For this review, take the finished solid that the model builds, in its own axes (mm). Round coordinates to 2 decimals unless told otherwise and drop trailing zeros. Write each loop counter-clockwise with the first axis right and the second up, starting at its lowest first coordinate (ties: lowest second). Pieces come first, ordered by that corner, then holes.
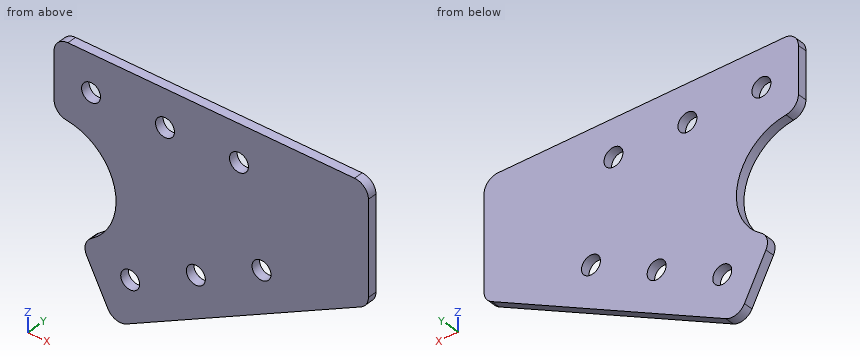
Autodesk Inventor part; units mm, degrees
ref_plane "YZ Plane" through (0, 0, 0) normal (1, 0, 0) x (0, 1, 0)
ref_plane "XZ Plane" through (0, 0, 0) normal (0, 1, 0) x (-1, 0, 0)
ref_plane "XY Plane" through (0, 0, 0) normal (0, 0, 1) x (1, 0, 0)
sketch "Sketch1" plane through (0, 0, 0) normal (0, 1, 0) x (-1, 0, 0)
  line L0 (0, 0) -> (0, -39.7058)
  line L1 (0, 0) -> (107.95, 0)
  line L2 (107.95, 0) -> (107.95, -25.4)
  line L3 (107.95, -25.4) -> (27.5892, -25.4)
  line L4 (0, -39.7058) -> (87.2373, -84.9409)
  line L5 (0, -3.175) -> (38.1, -3.175) construction
  line L6 (38.1, -3.175) -> (38.1, -22.225) construction
  line L7 (38.1, -22.225) -> (0, -22.225) construction
  line L8 (0, -22.225) -> (0, -3.175) construction
  circle A0 centre (44.45, -12.7) radius 3.2512
  circle A1 centre (69.85, -12.7) radius 3.2512
  circle A2 centre (95.25, -12.7) radius 3.2512
  line L9 (27.5892, -25.4) -> (0, -18.6724) construction
  circle A3 centre (36.7113, -44.4359) radius 3.2512
  circle A4 centre (59.2601, -56.1281) radius 3.2512
  circle A5 centre (81.809, -67.8203) radius 3.2512
  line L10 (27.5892, -25.4) -> (98.9296, -62.392)
  line L11 (81.809, -67.8203) -> (93.0834, -73.6665) construction
  line L12 (98.9296, -62.392) -> (87.2373, -84.9409)
  point P0 (38.1, -12.7)
  dimension "d0" = 39.7058
  dimension "d1" = 25.4
  dimension "d2" = 27.5892
  dimension "d4" = 107.95
  dimension "d5" = 19.05
  dimension "d6" = 3.175
  dimension "d7" = 38.1
  dimension "d8" = 6.5024
  dimension "d9" = 6.35
  dimension "d10" = 25.4
  dimension "d11" = 25.4
  dimension "d14" = 62.592
  dimension "d15" = 12.7
  dimension "d16" = 27.408
  dimension "d17" = 166.296
extrude "Extrusion1" add sketch "Sketch1" along normal blind 3.175
fillet "Fillet1" radius 19.05 1 edges at (-27.5892, 1.5875, -25.4)
fillet "Fillet2" radius 4.7625 6 edges at (-107.95, 1.5875, 0) (-107.95, 1.5875, -25.4) (-98.9296, 1.5875, -62.392) (-87.2373, 1.5875, -84.9409) (0, 1.5875, 0) (0, 1.5875, -39.7058)
properties part number "STRU_018_AngleBracket_62" material "Aluminum 6061"
(1) For line 1 along Z through (x, y) = (-95.25, 1); line 2 along X through (y, z) = (1.45, -65); line 3 along X through (y, z) = (2.5, -53.5), list the stretches that pass through material, from the lowest coordinate up.
Geometry check:
line 1: z = -69.49 to -60.37, -28.53 to -15.95, -9.45 to 0
line 2: x = -97.28 to -83.43, -80.19 to -48.78
line 3: x = -88.95 to -61.17, -57.35 to -26.6
(2) We need section A-A, the plane z = -12.7. Give the boundary of the cut face in (x, y) (3 decimals), and give its area (3 significant figures).
Geometry check:
outline: (-107.95, 0) - (-98.501, 0) - (-98.501, 3.175) - (-107.95, 3.175) - close; (-91.999, 0) - (-73.101, 0) - (-73.101, 3.175) - (-91.999, 3.175) - close; (-66.599, 0) - (-47.701, 0) - (-47.701, 3.175) - (-66.599, 3.175) - close; (-41.199, 0) - (0, 0) - (0, 3.175) - (-41.199, 3.175) - close
area: 281 mm2
(3) We need section B-B, the plane x = -58. Give the boundary of the cut face in (y, z) (1 decimal).
Geometry check:
outline: (0, -69.8) - (3.2, -69.8) - (3.2, -59.1) - (0, -59.1) - close; (0, -53.1) - (3.2, -53.1) - (3.2, 0) - (0, 0) - close
(4) We need section C-C, the plane x = -44.45. Give the boundary of the cut face in (y, z) (3 decimals).
Geometry check:
outline: (0, -62.754) - (3.175, -62.754) - (3.175, -15.951) - (0, -15.951) - close; (0, -9.449) - (3.175, -9.449) - (3.175, 0) - (0, 0) - close
(5) For pin 1 Ø1.5 at (y, z) = (2.5, -55) entering from +X; pin 2 Ø1.5 at (x, y) = (-45.5, 1.5) entering from -Z, all flat-tipped, find the tip position at first contact; note any pin that passes through.
Geometry check:
pin 1: stops at x = -28.05
pin 2: stops at z = -63.69
(6) We need section D-D, the plane z = -27. Give the boundary of the cut face in (x, y) (3 decimals).
Geometry check:
outline: (-98.07, 0) - (0, 0) - (0, 3.175) - (-98.07, 3.175) - close
